```python
from build123d import *

# Parameters (mm, degrees)
ESQUISSE1_R        = 45
BOSS_EXTRU_8_DEPTH = 700
BOSS_EXTRU_9_START = 60
ESQUISSE6_R        = 45
BOSS_EXTRU_9_DEPTH = 60


with BuildPart() as part:
    # Esquisse1 → Boss.-Extru.8 (new body)
    with BuildSketch(Plane.XY):
        with Locations((-5.0559795, 0.208317709)):
            Circle(ESQUISSE1_R)
    extrude(amount=BOSS_EXTRU_8_DEPTH)

    # Esquisse6 → Boss.-Extru.9 (add)
    # profile 1 of 4: a face of its own
    with BuildSketch(Plane(origin=(0, 0, 0), x_dir=(-1, 0, 0), z_dir=(0, 0, -1)).offset(BOSS_EXTRU_9_START)):
        Polygon((4.92504327, 101.776708668), (106.333278208, 0.8368395), (4.896305663, -101.070805399), (-96.511929276, -0.13093623), align=None)
        with Locations((5.0559795, 0.208317709)):
            Circle(ESQUISSE6_R, mode=Mode.SUBTRACT)
    # profile 2 of 4: a face of its own
    with BuildSketch(Plane(origin=(0, 0, 0), x_dir=(-1, 0, 0), z_dir=(0, 0, -1)).offset(BOSS_EXTRU_9_START)):
        Polygon((5.0559795, 45.208317709), (49.764887249, 0.705903269), (4.765369432, -44.50241444), (-39.943538316, 0), align=None)
    # profile 3 of 4: a face of its own
    with BuildSketch(Plane(origin=(0, 0, 0), x_dir=(-1, 0, 0), z_dir=(0, 0, -1)).offset(BOSS_EXTRU_9_START)):
        with BuildLine():
            ThreePointArc((50.0559795, 0.208317709), (36.875784654, 32.028122862), (5.0559795, 45.208317709))
            Line((5.0559795, 45.208317709), (49.764887249, 0.705903269))
            Line((49.764887249, 0.705903269), (4.765369432, -44.50241444))
            Line((4.765369432, -44.50241444), (-39.943538316, 0))
            ThreePointArc((-39.943538316, 0), (5.160138634, -44.791561745), (50.0559795, 0.208317709))
        make_face()
    # profile 4 of 4: a face of its own
    with BuildSketch(Plane(origin=(0, 0, 0), x_dir=(-1, 0, 0), z_dir=(0, 0, -1)).offset(BOSS_EXTRU_9_START)):
        with BuildLine():
            Line((-39.943538316, 0), (5.0559795, 45.208317709))
            ThreePointArc((5.0559795, 45.208317709), (-26.837392044, 31.954385994), (-39.943538316, 0))
        make_face()
    extrude(amount=-BOSS_EXTRU_9_DEPTH)


solid = part.part
```
Check sheet for the modelled part. Datum: model origin and axes. Units: mm. A direction names the side the tool comes from. Give positions to 0.01 mm unless a question says otherwise; leave off trailing zeros. Order: outer loops, then holes, each group sorted by start corner. A loop starts at its lowest first (then second) coordinate and runs counter-clockwise, first axis right, second up. Notation, with made-up numbers: M 57.5,-13 L 90.5,-13 A33 ccw 90.5,23 Z; hole C 42,-29 d9. An arc over 180 degrees is marked long. Answer in a Markdown table with one row per item.
1) Cross-section at D-D, the plane y = -70. Enter the section's corners in (x, z), plus the area to 3 significant figures.
Filled sheet:
| item | result |
|---|---|
| outline | M -35.82,-60 L 26.32,-60 L 26.32,0 L -35.82,0 Z |
| area | 3,730 mm2 |
2) Cross-section at C-C, the plane z = 222. Enter the section's corners in (x, y), plus the area to 3 significant figures.
Filled sheet:
| item | result |
|---|---|
| outline | C -5.06,0.21 d90 |
| area | 6,360 mm2 |
3) Access from +Z, -Z, +X, -X, +Y, -Y to the whole of each face (thin tool, end or side, straight path). Record for faces 1 (the flat face through (-6, 1, 700)), 2 (the cylindrical face through (19.14, 38.15, 345.1)).
Filled sheet:
| item | result |
|---|---|
| face 1 | +Z, +X, -X, +Y, -Y |
| face 2 | +Z |
4) Cross-section at A-A, the plane y = 17. Enter the section's corners in (x, z).
Filled sheet:
| item | result |
|---|---|
| outline | M -90.1,-60 L 79.46,-60 L 79.46,0 L 36.69,0 L 36.69,700 L -46.81,700 L -46.81,0 L -90.1,0 Z |
5) Cross-section at B-B, the plane x = -29. Enter the section's corners in (y, z), plus the area to 3 significant figures.
Filled sheet:
| item | result |
|---|---|
| outline | M -76.86,-60 L 77.81,-60 L 77.81,0 L 38.31,0 L 38.31,700 L -37.89,700 L -37.89,0 L -76.86,0 Z |
| area | 62,600 mm2 |
6) Gauge pin test, flat ends, axial feed: P1, Ø8, axis at x = -20, z = 349.5, coming from the +Y side; P2, Ø2, axis at x = -10.5, z = 606, coming from the +Y side; P3, Ø6, axis at x = -44, y = -54.5, coming from the +Z side. Record the tip position at first contact, or that the pin passes through.
Filled sheet:
| item | result |
|---|---|
| P1 | stops at y = 43.86 |
| P2 | stops at y = 44.99 |
| P3 | stops at z = 0 |
7) Thickness scan on L1, parallel to Z at x = 3, y = -73.5; L2, parallel to Y at x = 35, z = 554.5; L3, parallel to Y at x = -8, z = 363.5. Record the ranges inside material, lowest first. Write a range as [from, to].
Filled sheet:
| item | result |
|---|---|
| L1 | z = [-60, 0] |
| L2 | y = [-20.3, 20.71] |
| L3 | y = [-44.7, 45.11] |
